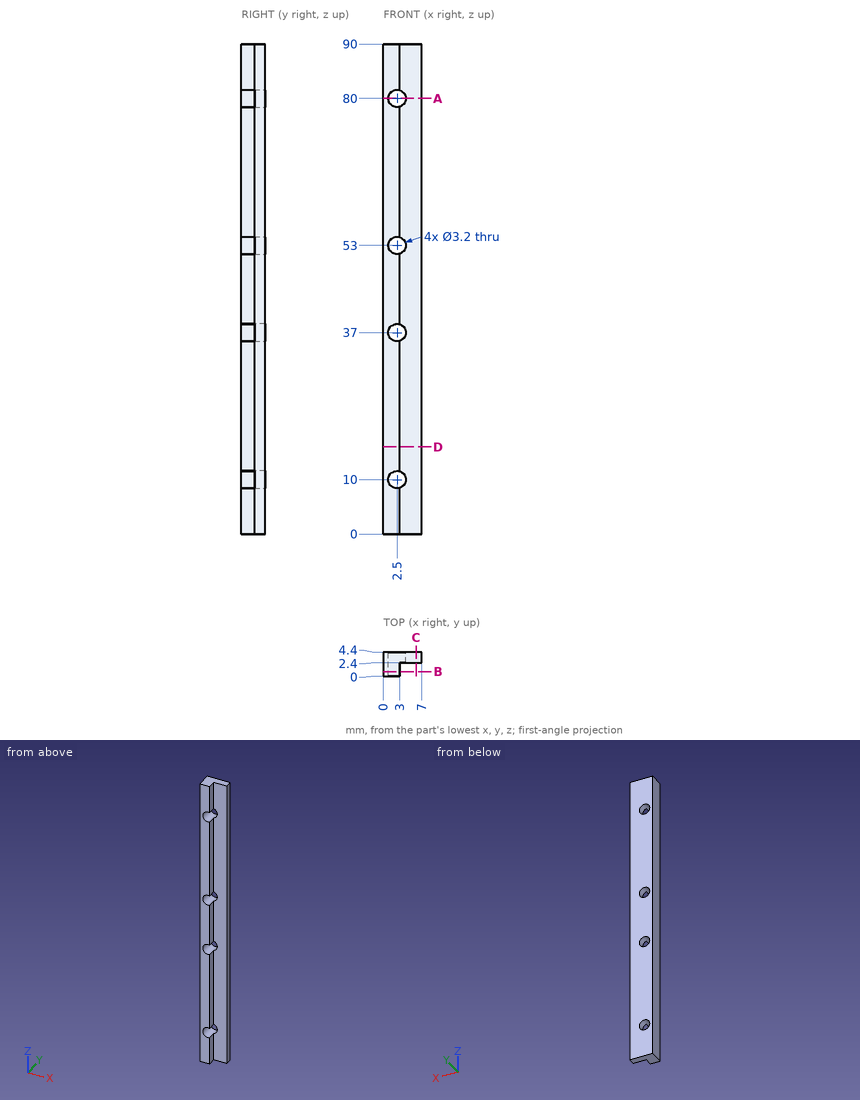
Geometry check sheet. Reference: drawing and pictorial views, mm from the part's lowest x, y, z. Give positions to 0.01 mm unless a question says otherwise; leave off trailing zeros. Order: outer loops, then holes, each group sorted by start corner. A loop starts at its lowest first (then second) coordinate and runs counter-clockwise, first axis right, second up. Notation, with made-up numbers: M 30,-8 L 66,-8 A21 ccw 66,13 Z; hole C -37.75,49 d4. An arc over 180 degrees is marked long. Answer in a Markdown table with one row per item. Add a question column.
Item 1: Section check C-C, the plane x = 6. Enter the section's corners in (y, z), and give its area (3 significant figures).
Item 2: Section check A-A, the plane z = 80. Enter the section's corners in (x, y).
Item 3: Gauge pin test, flat ends, axial feed: pin 1 (3.5 mm diameter, centred on x = 2.5, z = 37, fed in from +Y); pin 2 (0.7 mm diameter, centred on y = 1.5, z = 85.5, fed in from +X); pin 3 (1.2 mm diameter, centred on x = 5.5, z = 64.5, fed in from -Y). Record the tip position at first contact, or that the pin passes through.
Item 4: Scan lines: probe 1 along Z at (x, y) = (2.5, 2.9); probe 2 along Z at (x, y) = (2, 4.2); probe 3 along X at (y, z) = (3.4, 37). Record each from-to range of solid material in increasing order. Write a range as from..to.
Item 5: Section check B-B, the plane y = 0.8. Enter the section's corners in (x, z), and give its area (3 significant figures).
Item 6: Section check D-D, the plane z = 16. Enter the section's corners in (x, y), and give its area (3 significant figures).
Filled sheet:
| question | item | result |
|---|---|---|
| 1 | outline | M 2.4,0 L 4.4,0 L 4.4,90 L 2.4,90 Z |
| 1 | area | 180 mm^2 |
| 2 | outline | M 0,0 L 0.9,0 L 0.9,4.4 L 0,4.4 Z; M 4.1,2.4 L 7,2.4 L 7,4.4 L 4.1,4.4 Z |
| 3 | pin 1 | stops at y = 4.4 |
| 3 | pin 2 | stops at x = 3 |
| 3 | pin 3 | stops at y = 2.4 |
| 4 | probe 1 | z = 0..8.4, 11.6..35.4, 38.6..51.4, 54.6..78.4, 81.6..90 |
| 4 | probe 2 | z = 0..8.48, 11.52..35.48, 38.52..51.48, 54.52..78.48, 81.52..90 |
| 4 | probe 3 | x = 0..0.9, 4.1..7 |
| 5 | outline | M 0,0 L 3,0 L 3,8.48 A1.6 cw long 3,11.52 L 3,35.48 A1.6 cw long 3,38.52 L 3,51.48 A1.6 cw long 3,54.52 L 3,78.48 A1.6 cw long 3,81.52 L 3,90 L 0,90 Z |
| 5 | area | 248 mm^2 |
| 6 | outline | M 0,0 L 3,0 L 3,2.4 L 7,2.4 L 7,4.4 L 0,4.4 Z |
| 6 | area | 21.2 mm^2 |
